Answer from the drawing. Dimensions are ordinates in mm from the lowest x, y and z of the part. Give positions to 0.01 mm unless a question says otherwise; leave off trailing zeros. Write each loop counter-clockwise with the first axis right and the second up, starting at its lowest first coordinate (ties: lowest second). Pieces come first, ordered by that corner, then holes. Notation, with made-up numbers: (38, 76) -> (84, 76) arc R9 ccw to (84, 92) -> close; hole circle Ø11 at (67, -28.75). An arc over 180 degrees is marked (long way). Write item = value, one per line.
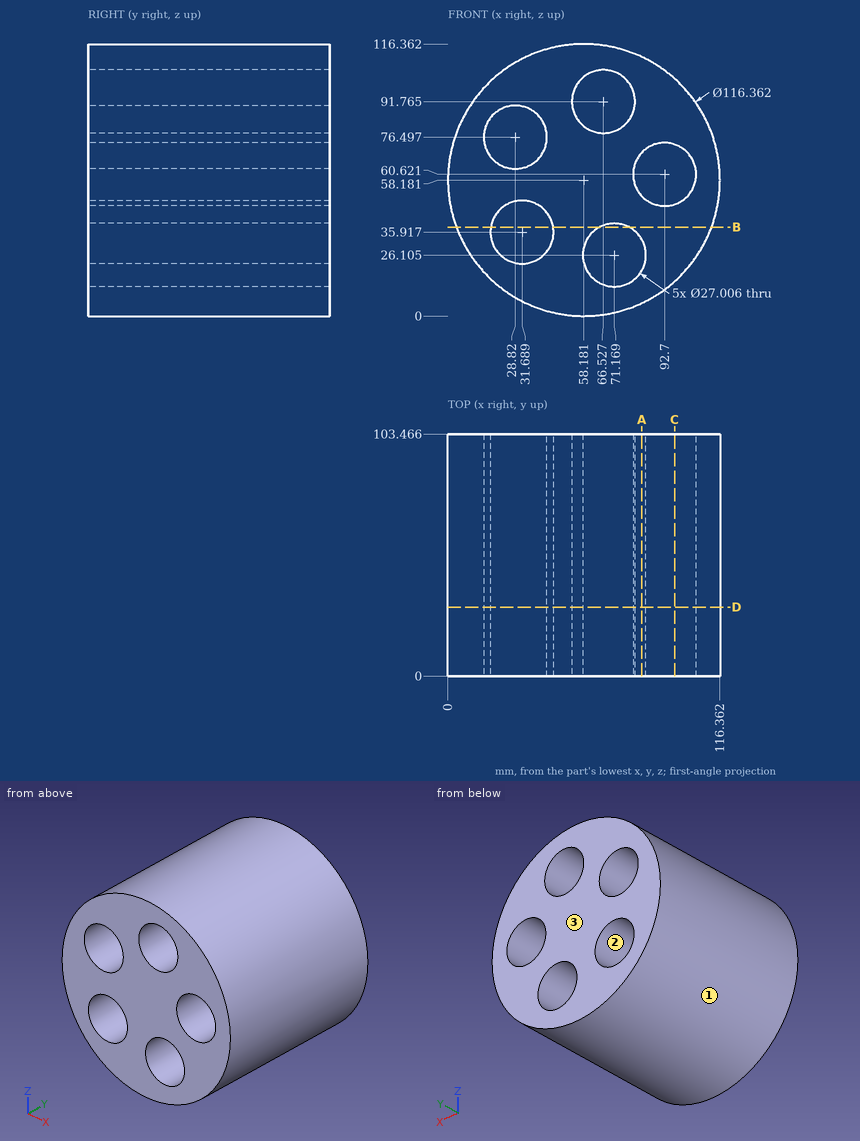
(1) The part is cut by section B-B on z = 38. Determine the outline of the cut face in (x, y), plus the area to 3 significant figures.
Checks:
outline = (3.61, 0) -> (18.35, 0) -> (18.35, 103.47) -> (3.61, 103.47) -> close; (45.03, 0) -> (64.78, 0) -> (64.78, 103.47) -> (45.03, 103.47) -> close; (77.56, 0) -> (112.75, 0) -> (112.75, 103.47) -> (77.56, 103.47) -> close
area = 7,210 mm²
(2) The part is cut by section D-D on y = 29.5. Determine the outline of the cut face in (x, z) (1 decimal), plus the area to 3 significant figures.
Checks:
outline = circle Ø116.4 at (58.2, 58.2); hole circle Ø27 at (28.8, 76.5); hole circle Ø27 at (31.7, 35.9); hole circle Ø27 at (66.5, 91.8); hole circle Ø27 at (71.2, 26.1); hole circle Ø27 at (92.7, 60.6)
area = 7,770 mm²
(3) The part is cut by section C-C on x = 97. Determine the outline of the cut face in (y, z), plus the area to 3 significant figures.
Checks:
outline = (0, 14.84) -> (103.47, 14.84) -> (103.47, 47.82) -> (0, 47.82) -> close; (0, 73.42) -> (103.47, 73.42) -> (103.47, 101.52) -> (0, 101.52) -> close
area = 6,320 mm²
(4) Given P1, Ø21.5, axis at x = 92.7, z = 60.62, coming from the -Y side; P2, Ø4, axis at y = 77, z = 83, coming from the +X side; P3, Ø1.5, axis at x = 104.5, y = 30, coming from the +Z side (1 decimal); P4, Ø8, axis at x = 28.5, y = 29, coming from the +Z side, each flat-ended and moving along its own axis, determine where each tip first touches the part or whether it passes through.
Checks:
P1 = through
P2 = 111.7
P3 = 94.4
P4 = 110.39
(5) The part is cut by section A-A on x = 83. Determine the outline of the cut face in (y, z) (1 decimal).
Checks:
outline = (0, 5.6) -> (103.5, 5.6) -> (103.5, 19.6) -> (0, 19.6) -> close; (0, 32.6) -> (103.5, 32.6) -> (103.5, 51.2) -> (0, 51.2) -> close; (0, 70) -> (103.5, 70) -> (103.5, 110.8) -> (0, 110.8) -> close
(6) Consider L1, parallel to X at y = 72, z = 64 (1 decimal); L2, parallel to Z at x = 78.5, y = 26.5 (1 decimal); L3, parallel to Z at x = 28.5, y = 39 (1 decimal). Determine where each line is inside the solid, lowest interval first.
Checks:
L1 = 0.3 to 23.7, 33.9 to 79.6, 105.8 to 116.1
L2 = 3.7 to 14.8, 37.4 to 85.5, 98 to 112.7
L3 = 8.1 to 22.8, 49 to 63, 90 to 108.2
(7) For a pull along X with two mould halves and no side action, classify the marked faces 1, 2 and 3 as released by +X, released by -X, zero draft, split by the parting line, or undercut.
Checks:
face_1 = split by the parting line
face_2 = undercut
face_3 = zero draft
